Source: three-view drawing plus pictorial views. Frame: mm from the lowest corner of the part. A direction names the side the tool comes from. Coordinates: 2 decimals unless noted, no trailing zeros. Write each loop counter-clockwise with the first axis right and the second up, starting at its lowest first coordinate (ties: lowest second). Pieces come first, ordered by that corner, then holes. Notation, with made-up numbers: (81.25, 68.5) - (117.25, 68.5) arc R27 cw to (117.25, 93.5) - close; hole circle Ø2 at (-6.5, 22.5). An arc over 180 degrees is marked (long way). One line per item, written item: value.
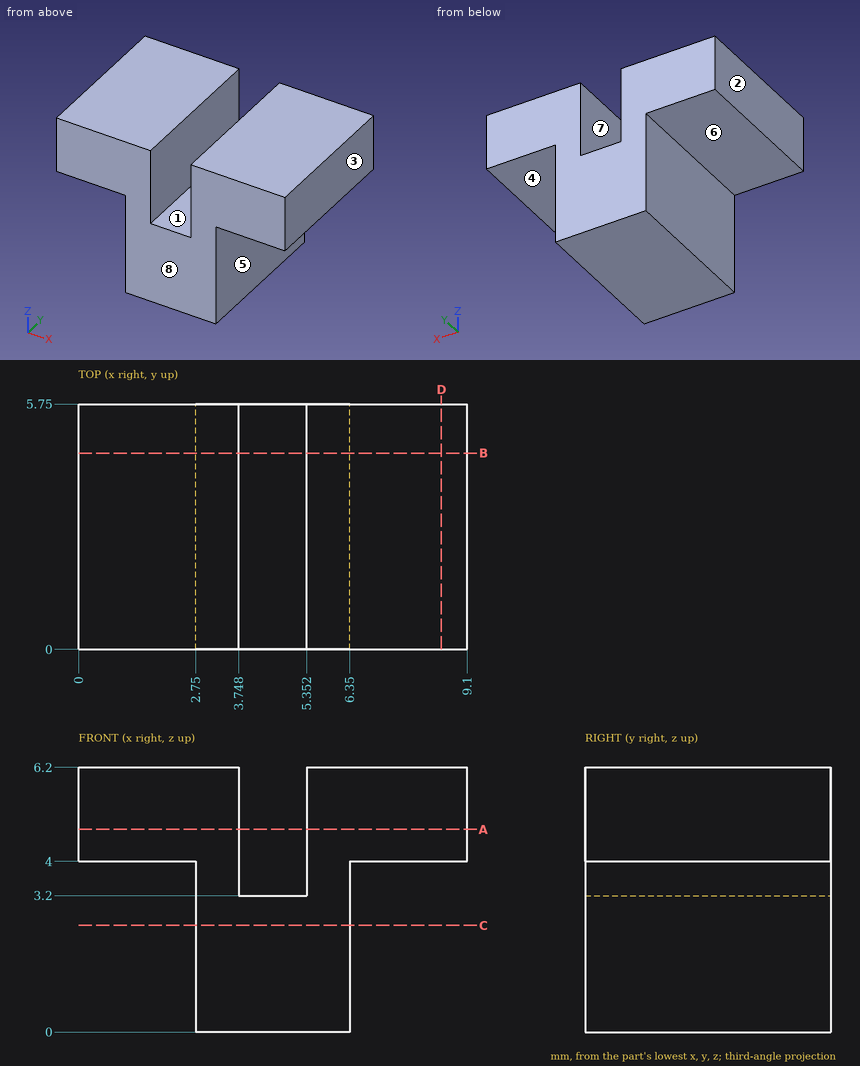
1) Reachability of the marked faces 5, 6, 7 and 8 from +Z, -Z, +X, -X, +Y, -Y: full face, straight path, thin tool, end or side. Return the list, or none.
Values found:
face 5: -Z, +X, +Y, -Y
face 6: -Z, -X, +Y, -Y
face 7: +Z, +Y, -Y
face 8: +Z, -Z, +X, -X, -Y
2) Section query D-D on x = 8.5. Output: boundary loops of the cut face in (y, z).
Values found:
outline: (0, 4) - (5.75, 4) - (5.75, 6.2) - (0, 6.2) - close
3) Section query C-C on z = 2.5. Output: boundary loops of the cut face in (x, y).
Values found:
outline: (2.75, 0) - (6.35, 0) - (6.35, 5.75) - (2.75, 5.75) - close
4) Contact query for flat-ended pins moving along their axis: P1, Ø1.4, axis at x = 8, y = 2.5, coming from the -Z side; P2, Ø2, axis at y = 2, z = 2.5, coming from the +X side; P3, Ø1.3, axis at x = 4.5, y = 2, coming from the +Z side. Output: stop coordinate, or through.
Values found:
P1: z = 4
P2: x = 6.35
P3: z = 3.2
5) Material intervals for line 1 (X direction, y = 2.05, z = 5.5); line 2 (X direction, y = 4.35, z = 2.75); line 3 (X direction, y = 4.1, z = 3.5), sorted ascending.
Values found:
line 1: 0 to 3.75, 5.35 to 9.1
line 2: 2.75 to 6.35
line 3: 2.75 to 3.75, 5.35 to 6.35
6) Section query B-B on y = 4.6. Output: boundary loops of the cut face in (x, z), then the cut area to 3 significant figures.
Values found:
outline: (0, 4) - (2.75, 4) - (2.75, 0) - (6.35, 0) - (6.35, 4) - (9.1, 4) - (9.1, 6.2) - (5.35, 6.2) - (5.35, 3.2) - (3.75, 3.2) - (3.75, 6.2) - (0, 6.2) - close
area: 29.6 mm2
7) Draft query along X for the marked faces 1, 2, 3 and 4. Return one class per face: released by +X, released by -X, zero draft, split by the parting line, or undercut.
Values found:
face 1: undercut
face 2: released by -X
face 3: released by +X
face 4: zero draft
8) Section query A-A on z = 4.75. Output: boundary loops of the cut face in (x, y).
Values found:
outline: (0, 0) - (3.75, 0) - (3.75, 5.75) - (0, 5.75) - close; (5.35, 0) - (9.1, 0) - (9.1, 5.75) - (5.35, 5.75) - close
